Here's how the part is built. I have some questions about the finished solid (model axes, mm). A direction names the side the tool comes from. Round coordinates to 2 decimals unless told otherwise and drop trailing zeros. Loops run counter-clockwise (first coordinate to the right, second up) from the corner with the lowest first, then second, coordinate; pieces in that order, holes last. Notation, with made-up numbers: (-38, -6.75) -> (-14, -6.75) arc R12 cw to (-14, -0.75) -> close; hole circle Ø7 at (89.25, -8). An arc over 180 degrees is marked (long way). Use one line per item in the form item = value. Start each with the question number.
Item 1: Thinking about a two-plate mould opening in Y: for faces 1 (the face through (5, 0, 4)), 2 (the face through (-5, 5, 9)), 3 (the face through (6.08, -4.96, 34.97)), 4 (the face through (-6.08, -6.77, 34.9)), which applies, released by +Y, released by -Y, zero draft, split by the parting line, or undercut?
Item 2: I'm going to push flat-ended pins straight in: pin 1 Ø5 at (y, z) = (0, 9) entering from +X; pin 2 Ø6.5 at (x, y) = (5.5, 0.5) entering from +Z; pin 3 Ø1.5 at (x, y) = (8.5, -5.5) entering from +Z; pin 4 Ø5 at (x, y) = (-4.5, 1) entering from +Z. Where does each tip first touch, or does it pass through?
Item 3: If we section it at C-C (x = -6.5): Write out the boundary of the cut face in (y, z) (1 decimal).
Item 4: For faces 5 (the face through (-2.13, 0, 11)), 6 (the face through (0, 0, 29)), 7 (the face through (5, 5, 9)), 8 (the face through (1.3, -3, 35)), which set-ups out of +Z, -Z, +X, -X, +Y, -Y let a thin tool reach every point of the face, with its end or its side?
Item 5: If we section it at D-D (z = 3): Write out the boundary of the cut face in (x, y), then the cut area to 3 significant figures.
Item 6: If I drill on L1, parallel to X at y = -2, z = 24; L2, parallel to Y at x = 9.25, z = 9; L3, parallel to Y at x = 0.25, z = 40, over which ranges is the centre line in solid material (lowest first)? Write a range as [from, to].
Item 7: If we section it at B-B (z = 9): Write out the boundary of the cut face in (x, y) (1 decimal).
Item 8: If we section it at A-A (x = 3.75): State how many separate pieces and enclosed holes the cut face has, then the cut area to 3 significant figures.
```python
from build123d import *

# Parameters (mm, degrees)
SKETCH1_R              = 1
BOSS_EXTRUDE1_DEPTH    = 11
SKETCH2_W              = 10
SKETCH2_H              = 6
BOSS_EXTRUDE2_DEPTH    = 4
CUT_EXTRUDE1_REACH     = 52.246
SKETCH3_R              = 1
FILLET1_R              = 2
SKETCH4_W              = 2.6
SKETCH4_H              = 8
CUT_EXTRUDE3_DEPTH     = 7
CUT_EXTRUDE4_START     = -8
CUT_EXTRUDE4_OUTLINE_W = 29
CUT_EXTRUDE4_OUTLINE_H = 14
CUT_EXTRUDE4_DEPTH     = 16
SKETCH5_3_R            = 1.5875
CUT_EXTRUDE5_DEPTH     = 12.5
SKETCH7_W              = 10
SKETCH7_H              = 10
SKETCH7_R              = 1.5875
BOSS_EXTRUDE3_DEPTH    = 5.87
BOSS_EXTRUDE4_START    = 5.865
SKETCH9_W              = 10
SKETCH9_H              = 10
SKETCH9_R              = 1.5875
BOSS_EXTRUDE4_DEPTH    = 5.865


# Read off the part's stored shape, not the designer's step: Cut-Extrude4
with BuildPart() as part:
    # Sketch1 → Boss-Extrude1 (new, symmetric)
    with BuildSketch(Plane(origin=(0, 0, 0), x_dir=(0, 0, -1), z_dir=(1, 0, 0))):
        with BuildLine():
            Line((-42.741088295, 3.837523613), (-35.598231152, -6.162476387))
            ThreePointArc((-35.598231152, -6.162476387), (-34.885927371, -6.778335285), (-33.970764209, -7))
            Line((-33.970764209, -7), (0, -7))
            Line((0, -7), (0, 7))
            Line((0, 7), (-41.113621352, 7))
            ThreePointArc((-41.113621352, 7), (-42.891956638, 5.915163162), (-42.741088295, 3.837523613))
        make_face()
        with Locations((-33.970764209, -5)):
            Circle(SKETCH1_R, mode=Mode.SUBTRACT)
    extrude(amount=BOSS_EXTRUDE1_DEPTH, both=True)

    # Sketch2 → Boss-Extrude2 (add)
    with BuildSketch(Plane(origin=(0, 7, 0), x_dir=(1, 0, 0), z_dir=(0, 1, 0))):
        with Locations((0, -44.113621352)):
            Rectangle(SKETCH2_W, SKETCH2_H)
    extrude(amount=-BOSS_EXTRUDE2_DEPTH)

    # Sketch3 → Cut-Extrude1 (cut, up to next)
    with BuildSketch(Plane(origin=(5, 0, 0), x_dir=(0, 0, -1), z_dir=(1, 0, 0)), mode=Mode.PRIVATE) as cut_extrude1_sk1:
        with Locations((-45.113621352, 5)):
            Circle(SKETCH3_R)
    cut_extrude1_tool1 = extrude(cut_extrude1_sk1.sketch, amount=-CUT_EXTRUDE1_REACH, mode=Mode.PRIVATE) & part.part
    add(cut_extrude1_tool1.solids().sort_by_distance((5, 5, 45.113621))[0], mode=Mode.SUBTRACT)

    # Fillet1
    fillet1_edges = [part.edges().sort_by_distance(p)[0] for p in [
        (0, 3, 47.113621352),
        (0, 7, 47.113621352),
    ]]
    fillet(fillet1_edges, radius=FILLET1_R - 0.0001)  # a hair under: the kernel refuses the full size

    # Sketch4 → Cut-Extrude3 (cut)
    with BuildSketch(Plane.XZ.offset(7)):
        with Locations((0, 35.598231152)):
            Rectangle(SKETCH4_W, SKETCH4_H)
    extrude(amount=-CUT_EXTRUDE3_DEPTH, mode=Mode.SUBTRACT)

    # Cut-Extrude4 outline → Cut-Extrude4 (cut)
    with BuildSketch(Plane.ZY.offset(CUT_EXTRUDE4_START)):
        with Locations((14.5, 0)):
            Rectangle(CUT_EXTRUDE4_OUTLINE_W, CUT_EXTRUDE4_OUTLINE_H)
    extrude(amount=CUT_EXTRUDE4_DEPTH, mode=Mode.SUBTRACT)

    # Sketch5<3> → Cut-Extrude5 (cut, symmetric)
    with BuildSketch(Plane.ZY):
        with Locations((9, 0)):
            Circle(SKETCH5_3_R)
    extrude(amount=CUT_EXTRUDE5_DEPTH, both=True, mode=Mode.SUBTRACT)

    # Sketch7 → Boss-Extrude3 (add)
    with BuildSketch(Plane(origin=(-8, 0, 0), x_dir=(0, 0, -1), z_dir=(1, 0, 0))):
        with Locations((-9, 0)):
            Rectangle(SKETCH7_W, SKETCH7_H)
        with Locations(Location((-9, 0, 0), (0, 0, 180))):
            Circle(SKETCH7_R, mode=Mode.SUBTRACT)
    extrude(amount=BOSS_EXTRUDE3_DEPTH)

    # Sketch9 → Boss-Extrude4 (add)
    with BuildSketch(Plane.ZY.offset(-8).offset(BOSS_EXTRUDE4_START)):
        with Locations((9, 0)):
            Rectangle(SKETCH9_W, SKETCH9_H)
        with Locations((9, 0)):
            Circle(SKETCH9_R, mode=Mode.SUBTRACT)
    extrude(amount=-BOSS_EXTRUDE4_DEPTH)


solid = part.part
```
Values found:
q1.face_1 = zero draft
q1.face_2 = released by +Y
q1.face_3 = undercut
q1.face_4 = released by -Y
q2.pin_1 = 11
q2.pin_2 = 46.64
q2.pin_3 = 36.61
q2.pin_4 = 46.44
q3.outline = (-7, 29) -> (7, 29) -> (7, 41.1) arc R2 ccw to (3.8, 42.7) -> (-6.2, 35.6) arc R2 ccw to (-7, 34) -> close; (-5, 4) -> (5, 4) -> (5, 14) -> (-5, 14) -> close; hole circle Ø2 at (-5, 34); hole circle Ø3.2 at (0, 9)
q4.face_5 = -Z, +Y, -Y
q4.face_6 = +Y, -Y
q4.face_7 = -Z, +Y
q4.face_8 = -Y
q5.outline = (-11, -7) -> (-8, -7) -> (-8, 7) -> (-11, 7) -> close; (8, -7) -> (11, -7) -> (11, 7) -> (8, 7) -> close
q5.area = 84.0 mm2
q6.L1 = [-11, -8], [8, 11]
q6.L2 = [-7, -1.59], [1.59, 7]
q6.L3 = [0, 7]
q7.outline = (-11, -7) -> (-8, -7) -> (-8, -5) -> (-2.1, -5) -> (-2.1, -1.6) -> (-11, -1.6) -> close; (-11, 1.6) -> (-2.1, 1.6) -> (-2.1, 5) -> (-8, 5) -> (-8, 7) -> (-11, 7) -> close; (2.1, -5) -> (8, -5) -> (8, -7) -> (11, -7) -> (11, -1.6) -> (2.1, -1.6) -> close; (2.1, 1.6) -> (11, 1.6) -> (11, 7) -> (8, 7) -> (8, 5) -> (2.1, 5) -> close
q8.separate_pieces = 2
q8.enclosed_holes = 3
q8.area = 252 mm2
